Read the model definition and answer for the solid it produces. Units are mm, in the model's axes. A direction names the side the tool comes from. Give positions to 0.01 mm unless a question says otherwise; leave off trailing zeros. Loops run counter-clockwise (first coordinate to the right, second up) from the corner with the lowest first, then second, coordinate; pieces in that order, holes last. Notation, with made-up numbers: (-40, 89) -> (-30, 89) arc R29 cw to (-30, 119) -> close; hole circle Ø9 at (25, -17.75). An arc over 180 degrees is marked (long way). One line per item, written item: value. Start each with the question number.
from build123d import *

# Parameters (mm, degrees)
SKETCH4_W           = 38.1
SKETCH4_H           = 76.2
SKETCH4_W_2         = 25.4
SKETCH4_H_2         = 63.5
BOSS_EXTRUDE1_DEPTH = 87.63


with BuildPart() as part:
    # Sketch4 → Boss-Extrude1 (new body)
    with BuildSketch(Plane.ZY.offset(152.4)):
        with Locations((6.35, 0)):
            Rectangle(SKETCH4_W, SKETCH4_H)
        with Locations((6.35, 0)):
            Rectangle(SKETCH4_W_2, SKETCH4_H_2, mode=Mode.SUBTRACT)
    extrude(amount=-BOSS_EXTRUDE1_DEPTH)


solid = part.part
Item 1: Determine the mould class of faces 3 (the flat face through (-109, -1, 25.4)), 4 (the flat face through (-109, 38.1, 6)), 5 (the flat face through (-109, 0, -6.35)), 6 (the flat face through (-109, 31.75, 6)) for opening direction Z: pulls with the +Z half, pulls with the -Z half, needs draft (parallel to the pull), parting line crosses it, or undercut.
Item 2: For faces 1 (the flat face through (-109, -1, -12.7)), 2 (the flat face through (-109, -31.75, 6)), determine the directions among +Z, -Z, +X, -X, +Y, -Y from which every point of the face is accessible in a straight line to the end or side of a thin tool.
Item 3: Section C-C, the plane z = 11 is taken. Determine the outline of the cut face in (x, y).
Item 4: Consider L1, parallel to Z at x = -70.5, y = 12; L2, parallel to Y at x = -82, z = -2. Determine where each line is inside the solid, lowest interval first. Write a range as [from, to].
Item 5: Section A-A, the plane y = -8 is taken. Determine the outline of the cut face in (x, z).
Item 6: A flat-ended cylindrical pin translates along its axis: pin 1 (6 mm diameter, centred on y = -1, z = -1, fed in from -X). Find the tip coordinate at first contact, or state that the pin passes through.
Item 7: Section B-B, the plane x = -96 is taken. Determine the outline of the cut face in (y, z).
Computed values:
1. face 3: pulls with the +Z half
1. face 4: needs draft
1. face 5: undercut
1. face 6: undercut
2. face 1: -Z, +X, -X, +Y, -Y
2. face 2: +X, -X
3. outline: (-152.4, -38.1) -> (-64.77, -38.1) -> (-64.77, -31.75) -> (-152.4, -31.75) -> close; (-152.4, 31.75) -> (-64.77, 31.75) -> (-64.77, 38.1) -> (-152.4, 38.1) -> close
4. L1: [-12.7, -6.35], [19.05, 25.4]
4. L2: [-38.1, -31.75], [31.75, 38.1]
5. outline: (-152.4, -12.7) -> (-64.77, -12.7) -> (-64.77, -6.35) -> (-152.4, -6.35) -> close; (-152.4, 19.05) -> (-64.77, 19.05) -> (-64.77, 25.4) -> (-152.4, 25.4) -> close
6. pin 1: through
7. outline: (-38.1, -12.7) -> (38.1, -12.7) -> (38.1, 25.4) -> (-38.1, 25.4) -> close; hole (-31.75, -6.35) -> (31.75, -6.35) -> (31.75, 19.05) -> (-31.75, 19.05) -> close
